from build123d import *

# Parameters (mm, degrees)
F0_W     = 50
F0_H     = 390
F1_DEPTH = 20
F3_DEPTH = 20.001
F4_W     = 15
F4_H     = 390
F5_DEPTH = 20.001


with BuildPart() as f1:
    # F0 (on Right) → F1 (new body)
    with BuildSketch(Plane.YZ):
        with Locations((-40.524636, 124.095061)):
            Rectangle(F0_W, F0_H)
    extrude(amount=F1_DEPTH)

    # F2 (on face) → F3 (cut, through all)
    with BuildSketch(Plane.YZ.offset(20)):
        with BuildLine():
            Line((-31.839951, -3.563652), (-65.524636, 51.735411))
            Line((-65.524636, 51.735411), (-65.524636, 13.706328))
            Line((-65.524636, 13.706328), (-49.812226, -12.088231))
            ThreePointArc((-49.812226, -12.088231), (-36.094721, -17.801029), (-31.839951, -3.563652))
        make_face()
        with BuildLine():
            Line((-31.839951, 76.436348), (-65.524636, 131.735411))
            Line((-65.524636, 131.735411), (-65.524636, 93.706328))
            Line((-65.524636, 93.706328), (-49.812226, 67.911769))
            ThreePointArc((-49.812226, 67.911769), (-36.094721, 62.198971), (-31.839951, 76.436348))
        make_face()
        with BuildLine():
            Line((-31.839951, 156.436348), (-65.524636, 211.735411))
            Line((-65.524636, 211.735411), (-65.524636, 173.706328))
            Line((-65.524636, 173.706328), (-49.812226, 147.911769))
            ThreePointArc((-49.812226, 147.911769), (-36.094721, 142.198971), (-31.839951, 156.436348))
        make_face()
        with BuildLine():
            Line((-31.839951, 236.436348), (-65.524636, 291.735411))
            Line((-65.524636, 291.735411), (-65.524636, 253.706328))
            Line((-65.524636, 253.706328), (-49.812226, 227.911769))
            ThreePointArc((-49.812226, 227.911769), (-36.094721, 222.198971), (-31.839951, 236.436348))
        make_face()
    extrude(amount=-F3_DEPTH, mode=Mode.SUBTRACT)

    # F4 (on face) → F5 (cut, through all)
    with BuildSketch(Plane.YZ.offset(20)):
        with Locations((-58.024636, 124.095061)):
            Rectangle(F4_W, F4_H)
    extrude(amount=-F5_DEPTH, mode=Mode.SUBTRACT)


solid = f1.part
Verification items for the finished model (mm, model axes). A direction names the side the tool comes from. Give positions to 0.01 mm unless a question says otherwise; leave off trailing zeros. Write each loop counter-clockwise with the first axis right and the second up, starting at its lowest first coordinate (ties: lowest second). Pieces come first, ordered by that corner, then holes. Notation, with made-up numbers: M 54.5,-27.5 L 59.5,-27.5 A10 cw 59.5,-9.5 Z; hole C 39,61 d9. An arc over 180 degrees is marked long. Put each result on its own line as item: value. Start each with the question number.
1. Set-up check for faces 5 (the face through (10, -50.525, 128)), 6 (the face through (10.14, -41.05, 11.56)): record each of +Z, -Z, +X, -X, +Y, -Y from which the full face is reachable in a straight line by a thin tool's end or side.
2. Section check B-B (y = -37.5). Record the cut outline in (x, z), and give its area (3 significant figures).
3. Section check C-C (z = 14). Record the cut outline in (x, y), and give its area (3 significant figures).
4. Section check A-A (x = 9.5). Record the cut outline in (y, z).
5. Section check D-D (z = 164). Record the cut outline in (x, y).
6. Scan lines: line 1 along Z through (x, y) = (11.75, -44.5); line 2 along Z through (x, y) = (13.5, -41); line 3 along Y through (x, z) = (12.75, 223.5). Record each from-to range of solid material in increasing order. Write a range as [from, to].
7. Go/stop test with flat-tipped pins: pin 1 Ø8 at (y, z) = (-25.5, 219.5) entering from -X; pin 2 Ø6 at (x, z) = (13.5, 77.5) entering from -Y. Record where each tip stops, or that it passes through.
8. Draft check along Y on faces 1 (the face through (10, -33, -70.905)), 2 (the face through (10.14, -36.31, -17.9)), 3 (the face through (10.14, -36.31, 142.1)), 4 (the face through (10.14, -41.05, 251.56)). Enter one of: +Y half, -Y half, draft (parallel to the pull), parting line (faces both ways), or undercut.
Answer list:
1. face 5: +Z, -Z, +X, -X, -Y
1. face 6: +X, -X, -Y
2. outline: M 0,-70.9 L 20,-70.9 L 20,-18.34 L 0,-18.34 Z; M 0,5.73 L 20,5.73 L 20,61.66 L 0,61.66 Z; M 0,85.73 L 20,85.73 L 20,141.66 L 0,141.66 Z; M 0,165.73 L 20,165.73 L 20,221.66 L 0,221.66 Z; M 0,245.73 L 20,245.73 L 20,319.1 L 0,319.1 Z
2. area: 5,870 mm2
3. outline: M 0,-42.54 L 20,-42.54 L 20,-15.52 L 0,-15.52 Z
3. area: 540 mm2
4. outline: M -50.52,-70.9 L -15.52,-70.9 L -15.52,319.1 L -50.52,319.1 L -50.52,267.11 L -31.84,236.44 A10 cw long -49.81,227.91 L -50.52,229.08 L -50.52,187.11 L -31.84,156.44 A10 cw long -49.81,147.91 L -50.52,149.08 L -50.52,107.11 L -31.84,76.44 A10 cw long -49.81,67.91 L -50.52,69.08 L -50.52,27.11 L -31.84,-3.56 A10 cw long -49.81,-12.09 L -50.52,-10.92 Z
5. outline: M 0,-36.45 L 20,-36.45 L 20,-15.52 L 0,-15.52 Z
6. line 1: [-70.9, -17.88], [17.22, 62.12], [97.22, 142.12], [177.22, 222.12], [257.22, 319.1]
6. line 2: [-70.9, -18.75], [11.47, 61.25], [91.47, 141.25], [171.47, 221.25], [251.47, 319.1]
6. line 3: [-50.52, -46.72], [-34.04, -15.52]
7. pin 1: x = 0
7. pin 2: y = -34.32
8. face 1: draft
8. face 2: undercut
8. face 3: undercut
8. face 4: -Y half
